from build123d import *

# Parameters (mm, degrees)
F1_DEPTH  = 5
F3_DEPTH  = 18
F4_R      = 8
F6_DEPTH  = 20
F8_DEPTH  = 69
F10_DEPTH = 2


with BuildPart() as f1:
    # F0 (on Front) → F1 (new body)
    with BuildSketch(Plane.XZ):
        with BuildLine():
            Line((-136.909834867, 61), (-136.909834867, -2.5))
            Line((-136.909834867, -2.5), (156.2171810981, -0.1359955775))
            ThreePointArc((156.2171810981, -0.1359955775), (168.1492733016, 4.8912054731), (173.0800843239, 16.863451604))
            Line((173.0800843239, 16.863451604), (173.0800843239, 41.636548396))
            ThreePointArc((173.0800843239, 41.636548396), (168.1492733016, 53.6087945269), (156.2171810981, 58.6359955775))
            Line((156.2171810981, 58.6359955775), (-136.909834867, 61))
        make_face()
    extrude(amount=F1_DEPTH)

    # F2 (on face) → F3 (join)
    with BuildSketch(Plane.XZ.offset(5)):
        with BuildLine():
            Line((169.0800786018, 16.863451604), (169.0800786018, 41.636548396))
            ThreePointArc((169.0800786018, 41.636548396), (165.309460068, 50.7917914076), (156.1849229874, 54.6361199305))
            Line((156.1849229874, 54.6361199305), (-134.909838438, 54.75))
            Line((-134.909838438, 54.75), (-134.909838438, 3.75))
            Line((-134.909838438, 3.75), (156.1849229874, 3.8638800695))
            ThreePointArc((156.1849229874, 3.8638800695), (165.309460068, 7.7082085924), (169.0800786018, 16.863451604))
        make_face()
    extrude(amount=F3_DEPTH)

    # F4
    f4_edges = [f1.edges().sort_by_distance(p)[0] for p in [
        (10.637542, -23, 54.69306),
        (165.30946, -23, 50.791791),
        (169.080079, -23, 29.25),
        (165.30946, -23, 7.708209),
        (10.637542, -23, 3.80694),
    ]]
    fillet(f4_edges, radius=F4_R)

    # F5 (on face) → F6 (join)
    with BuildSketch(Plane.XZ.offset(5)):
        Polygon((-134.909838438, 3.75), (-134.909838438, 54.75), (-134.909838438, 60.983870472), (-136.909834867, 61), (-136.909834867, -2.5), (-134.909838438, -2.483870472), align=None)
    extrude(amount=F6_DEPTH)

    # F7 (on face) → F8 (join)
    with BuildSketch(Plane.YZ.offset(-134.909838438)):
        Polygon((-25, 60.983870472), (-25, -2.483870472), (-23, -2.483870472), (-23, 11.7500006122), (-23, 46.7499993878), (-23, 60.983870472), align=None)
    extrude(amount=F8_DEPTH)

    # F9 (on face) → F10 (cut)
    with BuildSketch(Plane.XZ.offset(25)):
        with BuildLine():
            Line((-65.909838438, -2.483870472), (-65.909838438, 29.25))
            add(Edge.make_bspline(
                [(-97.409834867, 12.75), (-65.909838438, 13.8700312972), (-65.9114625472, 23.4057943523), (-65.909838438, 29.25)],
                knots=[0, 0, 0, 0, 35.5598056101, 35.5598056101, 35.5598056101, 35.5598056101], degree=3))
            Line((-97.409834867, 12.75), (-111.909834867, 12.75))
            add(Edge.make_bspline(
                [(-133.7268669105, -2.483870472), (-131.7941304161, -2.4585653704), (-126.820763516, -1.9012974431), (-121.7865199651, 10.7168586647), (-115.048285193, 12.1039418314), (-111.909834867, 12.75)],
                knots=[0.04781603, 0.04781603, 0.04781603, 0.04781603, 0.2828665478, 0.6659825914, 1, 1, 1, 1], degree=3))
            Line((-133.7268669105, -2.483870472), (-65.909838438, -2.483870472))
        make_face()
        with BuildLine():
            Line((-65.909838438, 60.983870472), (-133.7268669105, 60.983870472))
            add(Edge.make_bspline(
                [(-133.7268669105, 60.983870472), (-131.7941304161, 60.9585653704), (-126.820763516, 60.4012974431), (-121.7865199651, 47.7831413353), (-115.048285193, 46.3960581686), (-111.909834867, 45.75)],
                knots=[0.04781603, 0.04781603, 0.04781603, 0.04781603, 0.2828665478, 0.6659825914, 1, 1, 1, 1], degree=3))
            Line((-111.909834867, 45.75), (-97.409834867, 45.75))
            add(Edge.make_bspline(
                [(-97.409834867, 45.75), (-65.909838438, 44.6299687028), (-65.9114625472, 35.0942056477), (-65.909838438, 29.25)],
                knots=[0, 0, 0, 0, 35.5598056101, 35.5598056101, 35.5598056101, 35.5598056101], degree=3))
            Line((-65.909838438, 29.25), (-65.909838438, 60.983870472))
        make_face()
    extrude(amount=-F10_DEPTH, mode=Mode.SUBTRACT)


solid = f1.part
For this review, take the finished solid that the model builds, in its own axes (mm). A direction names the side the tool comes from. Coordinates: 2 decimals unless noted, no trailing zeros. Loops run counter-clockwise (first coordinate to the right, second up) from the corner with the lowest first, then second, coordinate; pieces in that order, holes last. Notation, with made-up numbers: (0.5, -24) -> (7.5, -24) arc R16 ccw to (7.5, -3) -> close; hole circle Ø1 at (68, -11). An arc over 180 degrees is marked (long way). Write each question's results on one line, items separated by ' | '.
Q1. For pin 1 Ø5 at (y, z) = (-11, 29) entering from +X; pin 2 Ø8 at (x, y) = (-14.5, -14.5) entering from +Z; pin 3 Ø8 at (x, y) = (33, -8) entering from -Z, all flat-tipped, find the tip position at first contact; note any pin that passes through.
Taken from the geometry:
pin 1: x = 169.08 | pin 2: z = 54.7 | pin 3: z = -1.15
Q2. Mouldability with a two-part tool opening along X and no side actions: class faces 4 (the flat face through (-110, -25, 30)), 5 (the flat face through (173.08, -2, 29)), 6 (the flat face through (-130, -23, 52)) as +X half, -X half, draft (parallel to the pull), parting line (faces both ways), or undercut.
Taken from the geometry:
face 4: draft | face 5: +X half | face 6: undercut
Q3. Add section A-A, the plane y = -10. State the section outline as (x, z) points.
Taken from the geometry:
outline: (-136.91, -2.5) -> (-134.91, -2.48) -> (-134.91, 3.75) -> (156.18, 3.86) arc R13 ccw to (169.08, 16.86) -> (169.08, 41.64) arc R13 ccw to (156.18, 54.64) -> (-134.91, 54.75) -> (-134.91, 60.98) -> (-136.91, 61) -> close
Q4. To check wall thickness, follow line 1 along Y through (x, z) = (58.5, 47); line 2 along Z through (x, y) = (-110.5, -8); line 3 along X through (y, z) = (-9.5, 1). State the ranges of each line that lie inside material, in increasing order. Write a range as [from, to].
Taken from the geometry:
line 1: [-22.99, 0] | line 2: [3.76, 54.74] | line 3: [-136.91, -134.91]
Q5. Machinability: for faces 1 (the flat face through (169.08, -10, 29)), 2 (the flat face through (-134.91, -14, 57)), 3 (the cylindrical face through (165.2, -9.9, 7.6)), which of the approach directions +Z, -Z, +X, -X, +Y, -Y give a long, thin tool a straight path to every point of the face, cutting with its end or side? Answer none if there is none.
Taken from the geometry:
face 1: +Z, -Z, +X, -Y | face 2: +Z, +X | face 3: -Z, +X, -Y
